Job drawing, mm, ordinate dimensions from the low corner. One solid piece. A direction names the side the tool comes from. Give positions to 0.01 mm unless a question says otherwise; leave off trailing zeros. Loops run counter-clockwise (first coordinate to the right, second up) from the corner with the lowest first, then second, coordinate; pieces in that order, holes last. Notation, with made-up numbers: (69.5, 8.25) -> (91.5, 8.25) arc R9 ccw to (91.5, 24.25) -> close; hole circle Ø5 at (60, -7). An arc over 180 degrees is marked (long way). Answer as a JSON object with one key per item and string values. Group by question number.
Q1. Wall check: probe 1 along Y at (x, z) = (51.5, 17.5); probe 2 along Y at (x, z) = (74, 36.5); probe 3 along Z at (x, y) = (53.5, 5). Give the ranges that are in metal, low to high. Write a range as from..to.
Q2. Drop flat-ended pins along their axis: pin 1 (6 mm diameter, centred on x = 41, y = 9.5, fed in from -Z) (1 decimal); pin 2 (3 mm diameter, centred on x = 69, z = 54, fed in from -Y); pin 3 (10 mm diameter, centred on y = 22.5, z = 48.5, fed in from +X). Give the stop position or say it passes through.
Q3. Band-saw the part on C-C, the plane y = 12.25. Write the cut outline in (x, z), plus the area to 3 significant figures.
Q4. Tool access for the marked faces 1 and 2: list every direction of +Z, -Z, +X, -X, +Y, -Y with a clear straight run to the whole face (end or side of a thin tool).
Q5. Band-saw the part on B-B, the plane x = 54. Write the cut outline in (y, z) (1 decimal), plus the area to 3 significant figures.
Q6. Band-saw the part on D-D, the plane x = 31.5. Write the cut outline in (y, z) (1 decimal), plus the area to 3 significant figures.
Q7. Band-saw the part on A-A, the plane z = 13. Write the cut outline in (x, y) (1 decimal), plus the area to 3 significant figures.
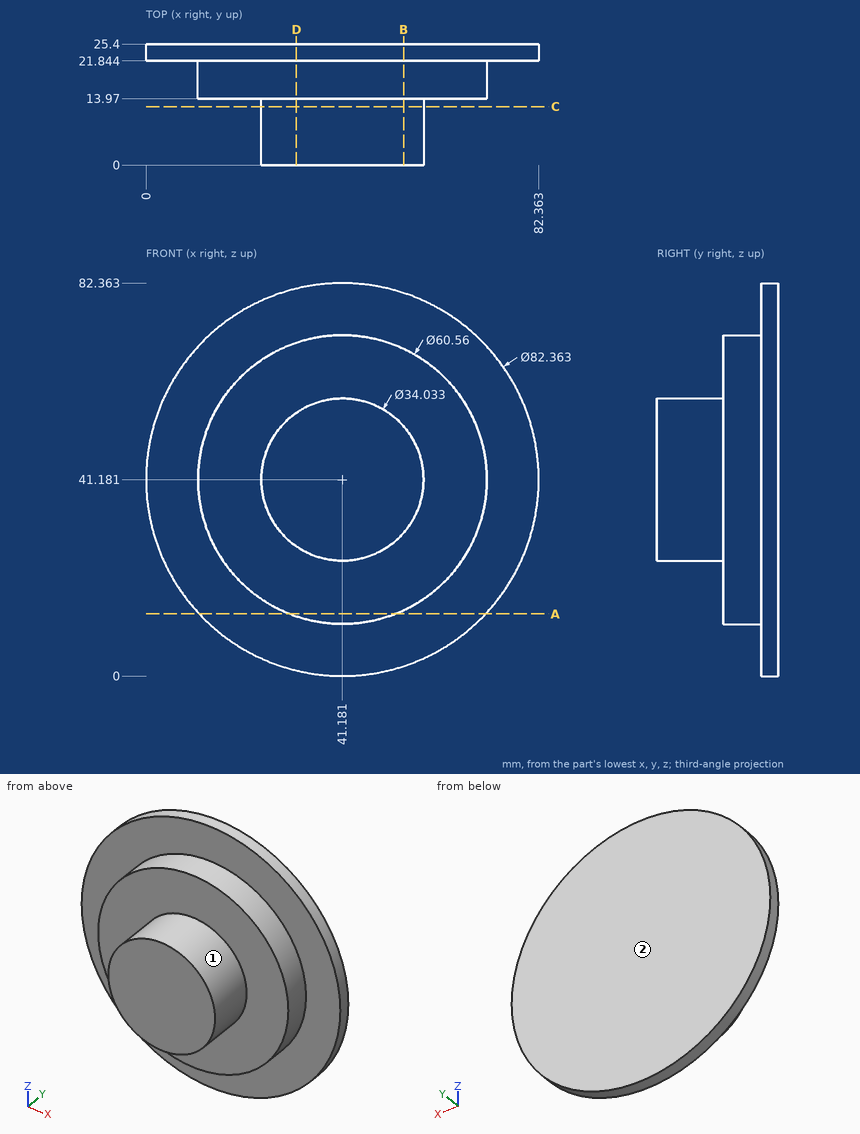
Worked answers:
{
 "1": {"probe 1": "13.97..25.4", "probe 2": "21.84..25.4", "probe 3": "29.44..52.92"},
 "2": {"pin 1": "z = 24.2", "pin 2": "y = 13.97", "pin 3": "x = 82.3"},
 "3": {"outline": "circle Ø34.03 at (41.18, 41.18)", "area": "910 mm2"},
 "4": {"face 1": "-Y", "face 2": "+Z, -Z, +X, -X, +Y"},
 "5": {"outline": "(0, 30) -> (14, 30) -> (14, 13.7) -> (21.8, 13.7) -> (21.8, 2) -> (25.4, 2) -> (25.4, 80.3) -> (21.8, 80.3) -> (21.8, 68.6) -> (14, 68.6) -> (14, 52.4) -> (0, 52.4) -> close", "area": "1,020 mm2"},
 "6": {"outline": "(0, 27.2) -> (14, 27.2) -> (14, 12.5) -> (21.8, 12.5) -> (21.8, 1.2) -> (25.4, 1.2) -> (25.4, 81.2) -> (21.8, 81.2) -> (21.8, 69.9) -> (14, 69.9) -> (14, 55.2) -> (0, 55.2) -> close", "area": "1,130 mm2"},
 "7": {"outline": "(11.2, 21.8) -> (30.1, 21.8) -> (30.1, 14) -> (52.3, 14) -> (52.3, 21.8) -> (71.2, 21.8) -> (71.2, 25.4) -> (11.2, 25.4) -> close", "area": "388 mm2"}
}
